```python
from build123d import *

# Parameters (mm, degrees)
SKETCH1_W           = 2.5
SKETCH1_H           = 3
SKETCH1_W_2         = 0.5
SKETCH1_H_2         = 0.5
BOSS_EXTRUDE1_DEPTH = 2
SKETCH1_3_W         = 1
SKETCH1_3_H         = 2
BOSS_EXTRUDE2_DEPTH = 1.5
CHAMFER1_SIZE       = 0.25
SKETCH2_W           = 2.25
SKETCH2_H           = 2.5
SKETCH2_W_2         = 0.25
SKETCH2_H_2         = 0.25
CUT_EXTRUDE1_DEPTH  = 3.75
CUT_EXTRUDE2_REACH  = 7.339
SKETCH3_W           = 0.75
SKETCH3_H           = 0.75


with BuildPart() as part:
    # Sketch1 → Boss-Extrude1 (new, symmetric)
    with BuildSketch(Plane.XY):
        with Locations((-1.25, 1.5)):
            Rectangle(SKETCH1_W, SKETCH1_H)
        with Locations((-1.75, -0.25)):
            Rectangle(SKETCH1_W_2, SKETCH1_H_2)
    extrude(amount=BOSS_EXTRUDE1_DEPTH, both=True)

    # Sketch1_3 → Boss-Extrude2 (add, symmetric)
    with BuildSketch(Plane.XY):
        with Locations((-3, 1.15)):
            Rectangle(SKETCH1_3_W, SKETCH1_3_H)
    extrude(amount=BOSS_EXTRUDE2_DEPTH, both=True)

    # Chamfer1
    chamfer1_edges = [part.edges().sort_by_distance(p)[0] for p in [
        (-2.5, 2.15, 0),
        (-3.5, 0.15, 0),
    ]]
    chamfer(chamfer1_edges, length=CHAMFER1_SIZE)

    # Sketch2 → Cut-Extrude1 (cut)
    with BuildSketch(Plane.XY.offset(2)):
        with Locations((-1.125, 1.5)):
            Rectangle(SKETCH2_W, SKETCH2_H)
        with Locations((-0.725, 1.255)):
            Rectangle(SKETCH2_W_2, SKETCH2_H_2, mode=Mode.SUBTRACT)
    extrude(amount=-CUT_EXTRUDE1_DEPTH, mode=Mode.SUBTRACT)

    # Sketch3 → Cut-Extrude2 (cut, up to next)
    with BuildSketch(Plane(origin=(0, 3, 0), x_dir=(1, 0, 0), z_dir=(0, 1, 0)), mode=Mode.PRIVATE) as cut_extrude2_sk1:
        Polygon((-1.5, -2), (0, -2), (0, -0.5), (-1.5, -0.5), (-1.5, -1.25), align=None)
    cut_extrude2_tool1 = extrude(cut_extrude2_sk1.sketch, amount=-CUT_EXTRUDE2_REACH, mode=Mode.PRIVATE) & part.part
    # Sketch3 → Cut-Extrude2 (cut, up to next)
    with BuildSketch(Plane(origin=(0, 3, 0), x_dir=(1, 0, 0), z_dir=(0, 1, 0)), mode=Mode.PRIVATE) as cut_extrude2_sk2:
        with Locations((-1.875, -1.625)):
            Rectangle(SKETCH3_W, SKETCH3_H)
    cut_extrude2_tool2 = extrude(cut_extrude2_sk2.sketch, amount=-CUT_EXTRUDE2_REACH, mode=Mode.PRIVATE) & part.part
    add(cut_extrude2_tool1.solids().sort_by_distance((-0.75, 3, 1.25))[0], mode=Mode.SUBTRACT)
    add(cut_extrude2_tool2.solids().sort_by_distance((-1.875, 3, 1.625))[0], mode=Mode.SUBTRACT)

    # Mirror1: part across plane


with BuildPart() as part_1:
    add(part.part)
    add(part.part.mirror(Plane(origin=(0, 0, 2), x_dir=(0, 0, 1), z_dir=(-1, 0, 0))))


solid = part_1.part
```
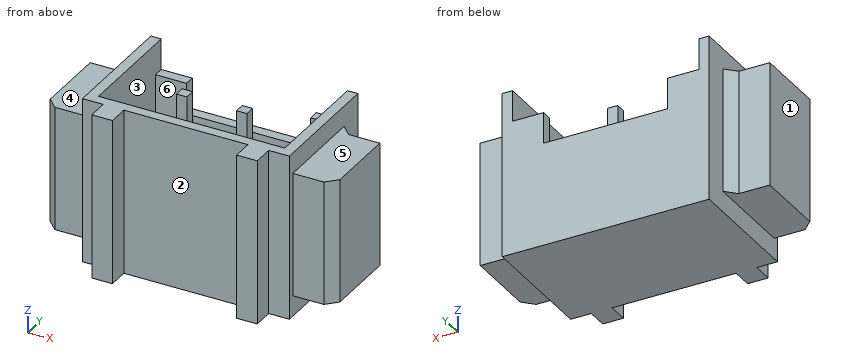
Here's how the part is built. I have some questions about the finished solid (model axes, mm). Face numbers are marked on the shaded views. A direction names the side the tool comes from. Round coordinates to 2 decimals unless told otherwise and drop trailing zeros. Write each loop counter-clockwise with the first axis right and the second up, starting at its lowest first coordinate (ties: lowest second). Pieces come first, ordered by that corner, then holes.
Q1. Please list where these lines run through material, in increasing order: probe 1 along X at (y, z) = (0.6, -0.3); probe 2 along X at (y, z) = (1.3, 0.8); probe 3 along X at (y, z) = (2.45, 1.75).
Q2. If we section it at C-C on y = 0.7: Write out the boundary of the cut face in (x, z), plus the area to 4 significant figures.
Q3. If we mould it in two halves opening along Y, with no side actions, what happens to the marked faces 1, 2 and 3? For each: +Y half, -Y half, draft (parallel to the pull), parting line (faces both ways), or undercut.
Q4. If we section it at B-B on z = 0.1: Give the number of separate pieces and of enclosed holes in the cut face, plus the area to 4 significant figures.
Q5. Which directions (+Z, -Z, +X, -X, +Y, -Y) give clear straight access to the entire face, cutting with the end or side of a thin tool? Please do the marked faces 4, 5 and 6.
Q6. If we section it at A-A on y = -0.1: Write out the boundary of the cut face in (x, z), plus the area to 3 significant figures.
Q7. Will these pins go through, and if not, where does the flat tip stop? P1, Ø1.5, axis at y = 2.5, z = 0.5, coming from the -X side; P2, Ø0.6, axis at x = -3, z = 0, coming from the +Y side; P3, Ø0.5, axis at x = 3, y = 1, coming from the -Z side.
Answer below:
1. probe 1: x = -3.5 to -2.25, 2.25 to 3.5
1. probe 2: x = -3.5 to -2.25, -0.85 to -0.6, 0.6 to 0.85, 2.25 to 3.5
1. probe 3: x = -2.5 to -2.25, 2.25 to 2.5
2. outline: (-3.5, -1.5) - (-2.5, -1.5) - (-2.5, -2) - (2.5, -2) - (2.5, -1.5) - (3.5, -1.5) - (3.5, 1.5) - (2.5, 1.5) - (2.5, 2) - (2.25, 2) - (2.25, -1.75) - (-2.25, -1.75) - (-2.25, 2) - (-2.5, 2) - (-2.5, 1.5) - (-3.5, 1.5) - close
2. area: 9.125 mm2
3. face 1: draft
3. face 2: -Y half
3. face 3: undercut
4. separate pieces: 3
4. enclosed holes: 1
4. area: 8.375 mm2
5. face 4: +Z, -X, +Y, -Y
5. face 5: +Z, +X, +Y, -Y
5. face 6: +Z
6. outline: (-2, -2) - (-1.5, -2) - (-1.5, 2) - (-2, 2) - close; (1.5, -2) - (2, -2) - (2, 2) - (1.5, 2) - close
6. area: 4.00 mm2
7. P1: stops at x = -3.5
7. P2: stops at y = 2.2
7. P3: stops at z = -1.5
